The model under review builds one solid part; all positions refer to its coordinate system, in mm. Round coordinates to 2 decimals unless told otherwise and drop trailing zeros. Order: outer loops, then holes, each group sorted by start corner. A loop starts at its lowest first (then second) coordinate and runs counter-clockwise, first axis right, second up.
```python
from build123d import *

# Parameters (mm, degrees)
SKETCH_1_W      = 117.92
SKETCH_1_H      = 55
SKETCH_1_R      = 1.1
SKETCH_1_R_2    = 1.5
EXTRUDE_1_DEPTH = 2


with BuildPart() as part:
    # 草图1 → 凸台-拉伸1 (new body)
    with BuildSketch(Plane(origin=(0, 0, 0), x_dir=(1, 0, 0), z_dir=(0, 1, 0))):
        with Locations((58.96, -27.5)):
            Rectangle(SKETCH_1_W, SKETCH_1_H)
        with Locations(Location((16.46, -2.97, 0), (0, 0, 270))):
            Circle(SKETCH_1_R, mode=Mode.SUBTRACT)
        with Locations(Location((30, -2.97, 0), (0, 0, 90))):
            Circle(SKETCH_1_R, mode=Mode.SUBTRACT)
        with Locations(Location((30, -23.03, 0), (0, 0, 270))):
            Circle(SKETCH_1_R, mode=Mode.SUBTRACT)
        with Locations(Location((16.46, -23.03, 0), (0, 0, 90))):
            Circle(SKETCH_1_R, mode=Mode.SUBTRACT)
        with Locations(Location((50, -5, 0), (0, 0, 270))):
            Circle(SKETCH_1_R_2, mode=Mode.SUBTRACT)
        with Locations(Location((107.92, -5, 0), (0, 0, 90))):
            Circle(SKETCH_1_R_2, mode=Mode.SUBTRACT)
        with Locations(Location((107.92, -27.8, 0), (0, 0, 270))):
            Circle(SKETCH_1_R_2, mode=Mode.SUBTRACT)
        with Locations(Location((50, -27.8, 0), (0, 0, 90))):
            Circle(SKETCH_1_R_2, mode=Mode.SUBTRACT)
        with BuildLine():
            Line((56.36, -47.5), (56.36, -42.5))
            ThreePointArc((56.36, -42.5), (58.96, -39.9), (61.56, -42.5))
            Line((61.56, -42.5), (61.56, -47.5))
            ThreePointArc((61.56, -47.5), (58.96, -50.1), (56.36, -47.5))
        make_face(mode=Mode.SUBTRACT)
        with BuildLine():
            ThreePointArc((95.019326342, -40.333675565), (95.32, -45), (95.019326342, -49.666324435))
            ThreePointArc((95.019326342, -49.666324435), (97.264150461, -52.578499683), (100.176325709, -50.333675565))
            ThreePointArc((100.176325709, -50.333675565), (100.52, -45), (100.176325709, -39.666324435))
            ThreePointArc((100.176325709, -39.666324435), (97.264150461, -37.421500317), (95.019326342, -40.333675565))
        make_face(mode=Mode.SUBTRACT)
        with BuildLine():
            ThreePointArc((22.900673658, -40.333675565), (20.655849539, -37.421500317), (17.743674291, -39.666324435))
            ThreePointArc((17.743674291, -39.666324435), (17.4, -45), (17.743674291, -50.333675565))
            ThreePointArc((17.743674291, -50.333675565), (20.655849539, -52.578499683), (22.900673658, -49.666324435))
            ThreePointArc((22.900673658, -49.666324435), (22.6, -45), (22.900673658, -40.333675565))
        make_face(mode=Mode.SUBTRACT)
    extrude(amount=EXTRUDE_1_DEPTH)


solid = part.part
```
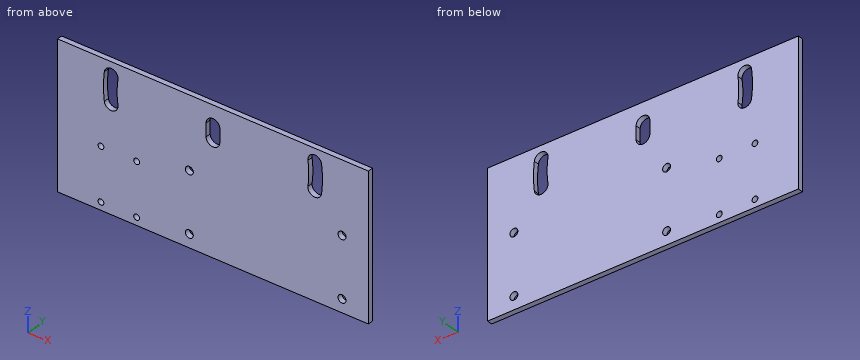
(1) Consider section C-C (y = 0.45). State how many separate pieces and enclosed holes the cut face has, and give its area (3 significant figures).
Data:
separate pieces: 1
enclosed holes: 11
area: 6,250 mm2
(2) To check wall thickness, follow probe 1 along X at (y, z) = (0.4, 27.8); probe 2 along Z at (x, y) = (108, 0.8); probe 3 along X at (y, z) = (1.25, 41). State the ranges of each line that lie inside material, in increasing order.
Data:
probe 1: x = 0 to 48.5, 51.5 to 106.42, 109.42 to 117.92
probe 2: z = 0 to 3.5, 6.5 to 26.3, 29.3 to 55
probe 3: x = 0 to 17.59, 22.82 to 56.84, 61.08 to 95.1, 100.33 to 117.92
(3) Consider section D-D (z = 45). Write out the cut boundary in (x, y).
Data:
outline: (0, 0) - (17.4, 0) - (17.4, 2) - (0, 2) - close; (22.6, 0) - (56.36, 0) - (56.36, 2) - (22.6, 2) - close; (61.56, 0) - (95.32, 0) - (95.32, 2) - (61.56, 2) - close; (100.52, 0) - (117.92, 0) - (117.92, 2) - (100.52, 2) - close
(4) Consider section A-A (z = 23.03). Write out the cut boundary in (x, y).
Data:
outline: (0, 0) - (15.36, 0) - (15.36, 2) - (0, 2) - close; (17.56, 0) - (28.9, 0) - (28.9, 2) - (17.56, 2) - close; (31.1, 0) - (117.92, 0) - (117.92, 2) - (31.1, 2) - close
(5) Consider section B-B (x = 50). Write out the cut boundary in (y, z), and give its area (3 significant figures).
Data:
outline: (0, 0) - (2, 0) - (2, 3.5) - (0, 3.5) - close; (0, 6.5) - (2, 6.5) - (2, 26.3) - (0, 26.3) - close; (0, 29.3) - (2, 29.3) - (2, 55) - (0, 55) - close
area: 98.0 mm2
